Read the model definition and answer for the solid it produces. Units are mm, in the model's axes. Face numbers are marked on the shaded views. Round coordinates to 2 decimals unless told otherwise and drop trailing zeros. Use one line per item in the form item = value. Start each with the question number.
1) For a pull along Y with two mould halves and no side action, classify the marked faces 1 and 2 as released by +Y, released by -Y, zero draft, split by the parting line, or undercut.
2) Consider line 1 along Y through (x, z) = (-46, 4); line 2 along Y through (x, z) = (-90, 2); line 3 along X through (y, z) = (29, 8.75). Determine where each line is inside the solid, lowest interval first. Write a range as from..to.
3) The part is cut by section A-A, the plane z = 6.25. Count the separate pieces of the cut face and the enclosed holes in it, plus the area to 3 significant figures.
4) Each of these flat-tipped pins is pushed along its axis until it touches: pin 1 (1 mm diameter, centred on x = -128.5, z = 5, fed in from +Y); pin 2 (3.5 mm diameter, centred on y = -31, z = 5.5, fed in from +X); pin 3 (5 mm diameter, centred on y = 34, z = 5.5, fed in from +X). Where does it stop, or does it pass through?
from build123d import *

# Parameters (mm, degrees)
BOSS_EXTRU_1_DEPTH      = 10
CONG_1_R                = 3
BOSS_EXTRU_2_DEPTH      = 2.7
CONG_2_R                = 2
ESQUISSE3_R             = 1
ENL_V_MAT_EXTRU_1_DEPTH = 20
ESQUISSE4_R             = 2
ENL_V_MAT_EXTRU_2_DEPTH = 2


with BuildPart() as part:
    # Model → Boss.-Extru.1 (new body)
    with BuildSketch(Plane.XY):
        Polygon((-26.464533767, 12.30154537), (75.33141454, 71.077500491), (143.246352653, 88.745859712), (161.383942986, 21.020985262), (100.854480283, 4.809102496), (-7.520422715, -57.858487698), (-179.373873722, -57.858487698), (-179.373873722, -50.687645053), (-179.373873722, 12.291034855), align=None)
        Polygon((-25.124548608, 7.301637465), (-174.373873722, 7.291378528), (-174.373873722, -50.687645053), (-174.373873722, -52.858487698), (-8.861972593, -52.858487698), (98.923133978, 9.468053786), (155.26069475, 24.557200291), (139.700811798, 82.657041562), (77.245358051, 66.408990356), align=None, mode=Mode.SUBTRACT)
    extrude(amount=BOSS_EXTRU_1_DEPTH)

    # Congé1
    cong_1_edges = [part.edges().sort_by_distance(p)[0] for p in [
        (75.33141454, 71.077500491, 5),
        (143.246352653, 88.745859712, 5),
        (161.383942986, 21.020985262, 5),
        (100.854480283, 4.809102496, 5),
        (-7.520422715, -57.858487698, 5),
        (-179.373873722, -57.858487698, 5),
        (-179.373873722, 12.291034855, 5),
        (-26.464533767, 12.30154537, 5),
    ]]
    fillet(cong_1_edges, radius=CONG_1_R)

    # Esquisse1 → Boss.-Extru.2 (add)
    with BuildSketch(Plane.XY):
        Polygon((-25.124548608, 7.301637465), (-174.373873722, 7.291378528), (-174.373873722, -50.687645053), (-174.373873722, -52.858487698), (-8.861972593, -52.858487698), (98.923133978, 9.468053786), (155.26069475, 24.557200291), (139.700811798, 82.657041562), (77.245358051, 66.408990356), align=None)
    extrude(amount=BOSS_EXTRU_2_DEPTH)

    # Congé2
    cong_2_edges = [part.edges().sort_by_distance(p)[0] for p in [
        (-101.821199292, 12.296365586, 0),
        (24.605627892, 41.788942262, 0),
        (108.044083383, 79.587840046, 0),
        (152.312387337, 54.893729991, 0),
        (129.861641055, 12.578223, 0),
        (46.843967712, -26.422377988, 0),
        (-92.349613182, -57.858487698, 0),
        (-179.373873722, -22.78362332, 0),
        (-178.495266971, 11.412488494, 0),
        (-178.495194066, -56.979808041, 0),
        (-7.547920203, -57.756003669, 0),
        (160.307894606, 21.642410085, 0),
        (142.628648998, 87.685066626, 0),
        (75.341794938, 71.05218052, 0),
        (-26.491925042, 12.40375087, 0),
        (100.86445313, 4.78504518, 0),
    ]]
    fillet(cong_2_edges, radius=CONG_2_R)

    # Esquisse3 → Enlèv. mat.-Extru.1 (cut)
    with BuildSketch(Plane.XY):
        with Locations(Location((158.201617013, 22.958080812, 0), (0, 0, 238.978237888))):
            Circle(ESQUISSE3_R)
        with Locations(Location((141.388472611, 85.534334234, 0), (0, 0, 154.767958728))):
            Circle(ESQUISSE3_R)
        with Locations(Location((76.500226548, 68.776582274, 0), (0, 0, 174.757995249))):
            Circle(ESQUISSE3_R)
        with Locations(Location((99.890442316, 7.071415488, 0), (0, 0, 236.208794577))):
            Circle(ESQUISSE3_R)
        with Locations(Location((-8.172352823, -55.275906246, 0), (0, 0, 215.632313771))):
            Circle(ESQUISSE3_R)
        with Locations(Location((-25.691359515, 9.920090126, 0), (0, 0, 154.730246838))):
            Circle(ESQUISSE3_R)
        with Locations(Location((-176.562127678, 9.920090126, 0), (0, 0, 215.825985053))):
            Circle(ESQUISSE3_R)
        with Locations(Location((-177.029598341, -55.275906246, 0), (0, 0, 155.328283389))):
            Circle(ESQUISSE3_R)
    extrude(amount=ENL_V_MAT_EXTRU_1_DEPTH, mode=Mode.SUBTRACT)

    # Esquisse4 → Enlèv. mat.-Extru.2 (cut)
    with BuildSketch(Plane(origin=(0, 0, 0), x_dir=(-1, 0, 0), z_dir=(0, 0, -1))):
        with Locations((177.029598341, -55.275906246)):
            Circle(ESQUISSE4_R)
        with Locations((176.562127678, 9.920090126)):
            Circle(ESQUISSE4_R)
        with Locations((25.691359515, 9.920090126)):
            Circle(ESQUISSE4_R)
        with Locations((-76.500226548, 68.776582274)):
            Circle(ESQUISSE4_R)
        with Locations((-141.388472611, 85.534334234)):
            Circle(ESQUISSE4_R)
        with Locations((-158.201617013, 22.958080812)):
            Circle(ESQUISSE4_R)
        with Locations((-99.890442316, 7.071415488)):
            Circle(ESQUISSE4_R)
        with Locations((8.172352823, -55.275906246)):
            Circle(ESQUISSE4_R)
    extrude(amount=-ENL_V_MAT_EXTRU_2_DEPTH, mode=Mode.SUBTRACT)


solid = part.part
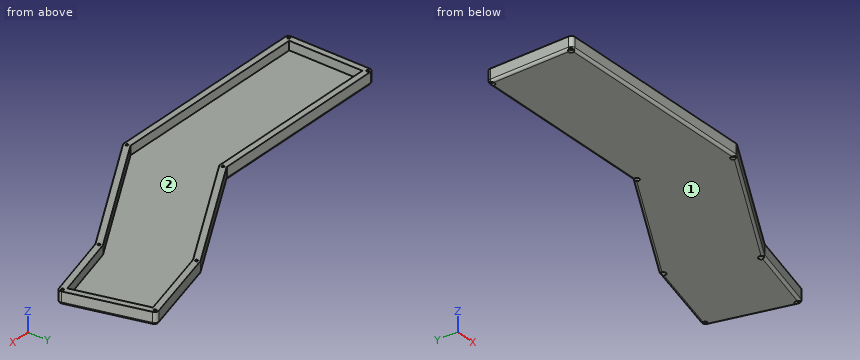
Geometry results:
q1.face_1 = zero draft
q1.face_2 = undercut
q2.line_1 = -57.86..-52.86, 7.3..12.3
q2.line_2 = -57.86..12.3
q2.line_3 = 2.46..12.46, 154.07..159.25
q3.separate_pieces = 1
q3.enclosed_holes = 9
q3.area = 4,070 mm2
q4.pin_1 = 12.29
q4.pin_2 = 41.95
q4.pin_3 = 158.58
